from build123d import *

# Parameters (mm, degrees)
F0_W           = 40.847726
F0_H           = 49.624716
F1_DEPTH       = 25.4
F2_R           = 5.08
F4_D           = 12.7
F4_CSINK_D     = 15.24
F4_CSINK_ANGLE = 49


with BuildPart() as f1:
    # F0 (on Front) → F1 (new body)
    with BuildSketch(Plane.XZ):
        with Locations((-42.006526, 12.353429)):
            Rectangle(F0_W, F0_H)
    extrude(amount=F1_DEPTH)

    # F2
    f2_edges = [f1.edges().sort_by_distance(p)[0] for p in [
        (-42.006526, -25.4, 37.165787),
        (-62.430389, -25.4, 12.353429),
        (-42.006526, -25.4, -12.458929),
        (-21.582663, -25.4, 12.353429),
        (-42.006526, 0, 37.165787),
        (-62.430389, 0, 12.353429),
        (-42.006526, 0, -12.458929),
        (-21.582663, 0, 12.353429),
    ]]
    fillet(f2_edges, radius=F2_R)

    # F4 (through all)
    with Locations(Plane.XZ.offset(25.4)):
        with Locations((-42.396232, 13.828625)):
            CounterSinkHole(F4_D / 2, F4_CSINK_D / 2, counter_sink_angle=F4_CSINK_ANGLE)


solid = f1.part
Model file for the job. Use its own axes, mm. Coordinates: 2 decimals unless noted, no trailing zeros. Loops run counter-clockwise (first coordinate to the right, second up) from the corner with the lowest first, then second, coordinate; pieces in that order, holes last. Notation, with made-up numbers: (50.5, -30) -> (67.5, -30) arc R7 ccw to (67.5, -19) -> close; hole circle Ø4 at (34.5, 13.5). An arc over 180 degrees is marked (long way). Use one line per item in the form item = value. Start each with the question number.
(1) Cut at C-C on y = -3.5. Give the cut face in (x, z).
(2) Pull direction X, two halves, no side cores. Call faces 1 (the cylindrical face through (-60.982, -1.528, 12.701)), 2 (the cylindrical face through (-41.57, -11.148, 20.125)), 3 (the flat face through (-21.583, -13, 12)), 4 (the cylindrical face through (-41.72, -1.53, 35.72)): pulls with the +X half, pulls with the -X half, needs draft (parallel to the pull), parting line crosses it, or undercut.
(3) Cut at A-A on z = 29.5. Give the cut face in (x, y), and give its area (3 significant figures).
(4) Probe probe 1 along Y at (x, z) = (-42, -7.5); probe 2 along X at (y, z) = (-18.5, 12); probe 3 along Z at (x, y) = (-48, -4.5). List the from-to ranges inside material, lowest first. Write a range as from..to.
(5) Cut at D-D on y = -8.5. Give the cut face in (x, z), and give its area (3 significant figures).
(6) Cut at B-B on x = -53.5. Give the cut face in (y, z).
Values:
q1.outline = (-62.18, -12.21) -> (-21.83, -12.21) -> (-21.83, 36.91) -> (-62.18, 36.91) -> close; hole circle Ø12.7 at (-42.4, 13.83)
q2.face_1 = pulls with the -X half
q2.face_2 = undercut
q2.face_3 = pulls with the +X half
q2.face_4 = needs draft
q3.outline = (-62.43, -20.32) arc R5.08 ccw to (-57.35, -25.4) -> (-26.66, -25.4) arc R5.08 ccw to (-21.58, -20.32) -> (-21.58, -5.08) arc R5.08 ccw to (-26.66, 0) -> (-57.35, 0) arc R5.08 ccw to (-62.43, -5.08) -> close
q3.area = 1,020 mm2
q4.probe_1 = -25.4..0
q4.probe_2 = -62.43..-48.48, -36.32..-21.58
q4.probe_3 = -12.43..10.84, 16.82..37.13
q5.outline = (-62.43, -12.46) -> (-21.58, -12.46) -> (-21.58, 37.17) -> (-62.43, 37.17) -> close; hole circle Ø12.7 at (-42.4, 13.83)
q5.area = 1,900 mm2
q6.outline = (-25.4, -7.38) arc R5.08 ccw to (-20.32, -12.46) -> (-5.08, -12.46) arc R5.08 ccw to (0, -7.38) -> (0, 32.09) arc R5.08 ccw to (-5.08, 37.17) -> (-20.32, 37.17) arc R5.08 ccw to (-25.4, 32.09) -> close
